```python
from build123d import *

# Parameters (mm, degrees)
SKETCH1_R                 = 4.7625
SKETCH1_W                 = 6.5278
SKETCH1_H                 = 6.5278
SKETCH1_H_2               = 6.348837221
BOSS_EXTRUDE1_DEPTH       = 6.35
F_6_CLEARANCE_HOLE1_D     = 3.7973
F_6_CLEARANCE_HOLE1_DEPTH = 12.7
F_6_CLEARANCE_HOLE1_TIP   = 1.140824014
SKETCH7_W                 = 6.35
SKETCH7_H                 = 6.1722
BOSS_EXTRUDE2_DEPTH       = 1.016
SKETCH8_W                 = 6.35
SKETCH8_H                 = 6.1722
BOSS_EXTRUDE3_DEPTH       = 1.016
SKETCH9_R                 = 1.5875
CUT_EXTRUDE1_DEPTH        = 161.894515133
CUT_EXTRUDE2_DEPTH        = 161.894515133


with BuildPart() as part:
    # Sketch1 → Boss-Extrude1 (new body)
    with BuildSketch(Plane(origin=(0, 0, 0), x_dir=(0, 0, -1), z_dir=(1, 0, 0))):
        Polygon((0, 0), (-14.664696837, 25.4), (-144.085303163, 25.4), (-158.75, 0), align=None)
        with Locations((-130.048, 12.7)):
            Circle(SKETCH1_R, mode=Mode.SUBTRACT)
        with Locations((-28.702, 12.7)):
            Circle(SKETCH1_R, mode=Mode.SUBTRACT)
        with Locations((-17.750796837, 12.6111)):
            Rectangle(SKETCH1_W, SKETCH1_H, mode=Mode.SUBTRACT)
        with Locations((-140.999203163, 12.70058139)):
            Rectangle(SKETCH1_W, SKETCH1_H_2, mode=Mode.SUBTRACT)
        with Locations((-79.4639, 12.7889)):
            Rectangle(SKETCH1_W, SKETCH1_H, mode=Mode.SUBTRACT)
    extrude(amount=BOSS_EXTRUDE1_DEPTH)

    # #6 Clearance Hole1
    with Locations(Plane(origin=(0, 25.4, 0), x_dir=(1, 0, 0), z_dir=(0, 1, 0))):
        with Locations((3.175, -79.375)):
            Hole(F_6_CLEARANCE_HOLE1_D / 2, depth=F_6_CLEARANCE_HOLE1_DEPTH)
            with Locations((0, 0, -(F_6_CLEARANCE_HOLE1_DEPTH + F_6_CLEARANCE_HOLE1_TIP / 2))):  # 118° drill point
                Cone(0, F_6_CLEARANCE_HOLE1_D / 2, F_6_CLEARANCE_HOLE1_TIP, mode=Mode.SUBTRACT)

    # Sketch7 → Boss-Extrude2 (add)
    with BuildSketch(Plane(origin=(0, 0, 0), x_dir=(-1, 0, 0), z_dir=(0, 0.499999999999998, -0.8660254037844397))):
        with Locations((-3.175, 19.893293675)):
            Rectangle(SKETCH7_W, SKETCH7_H)
    extrude(amount=BOSS_EXTRUDE2_DEPTH)

    # Sketch8 → Boss-Extrude3 (add)
    with BuildSketch(Plane(origin=(0, 68.740766425, 119.0625), x_dir=(1, 0, 0), z_dir=(0, 0.500000000000004, 0.8660254037844365))):
        with Locations((3.175, -59.481706325)):
            Rectangle(SKETCH8_W, SKETCH8_H)
    extrude(amount=BOSS_EXTRUDE3_DEPTH)

    # Sketch9 → Cut-Extrude1 (cut, through all)
    with BuildSketch(Plane(origin=(6.35, 0, 0), x_dir=(0, 0, -1), z_dir=(1, 0, 0))):
        with Locations((-151.13, 3.81)):
            Circle(SKETCH9_R)
        with Locations((-7.62, 3.81)):
            Circle(SKETCH9_R)
    extrude(amount=-CUT_EXTRUDE1_DEPTH, mode=Mode.SUBTRACT)

    # Sketch10 → Cut-Extrude2 (cut, through all)
    with BuildSketch(Plane(origin=(6.35, 0, 0), x_dir=(0, 0, -1), z_dir=(1, 0, 0))):
        Polygon((-90.0938, 7.366), (-90.0938, 17.550906382), (-115.628105199, 7.366), align=None)
        Polygon((-119.901628846, 7.849093618), (-94.367323648, 18.034), (-119.901628846, 18.034), align=None)
        Polygon((-68.834, 7.850665489), (-43.375663722, 18.034), (-68.834, 18.034), align=None)
        Polygon((-39.116, 7.366), (-39.116, 17.549334511), (-64.574336278, 7.366), align=None)
    extrude(amount=-CUT_EXTRUDE2_DEPTH, mode=Mode.SUBTRACT)


solid = part.part
```
Here's how the part is built. I have some questions about the finished solid (model axes, mm). A direction names the side the tool comes from. Coordinates: 2 decimals unless noted, no trailing zeros. Loops run counter-clockwise (first coordinate to the right, second up) from the corner with the lowest first, then second, coordinate; pieces in that order, holes last. Notation, with made-up numbers: (34.5, -18) - (50.5, -18) arc R28 cw to (50.5, 10) - close; hole circle Ø8 at (87.5, -39). An arc over 180 degrees is marked (long way). Return JSON: item names as keys, results as strings. Group by question number.
Item 1: If we section it at D-D on x = 2.25: State how many separate pieces and enclosed holes the cut face has, and give its area (3 significant figures).
Item 2: We'd pull the mould along Z, two halves only. Please class faces 1 (the face through (3.131, 7.176, 4.143)), 2 (the face through (3, 13, 76.2)), 3 (the face through (6.35, 7, 80)): +Z half, -Z half, draft (parallel to the pull), parting line (faces both ways), or undercut.
Item 3: Will these pins go through, and if not, where does the flat tip stop? P1, Ø3, axis at x = 3, z = 18.5, coming from the -Y side; P2, Ø1.9, axis at x = 4, y = 14, coming from the +Z side; P3, Ø3, axis at x = 2.5, y = 13, coming from the +Z side; P4, Ø3, axis at x = 2.5, y = 11.5, coming from the +Z side.
Item 4: If we section it at A-A on y = 3.81: Write out the boundary of the cut face in (x, z).
Item 5: On a 3-axis mill with a long thin cutter (end or side, diameter ignored), from which of +Z, -Z, +X, -X, +Y, -Y can I reach the whole of each face in a straight line? I mean faces 4 (the face through (5, 25.4, 78)), 5 (the face through (3, 7.366, 52)). Say none if no direction works.
Item 6: If we section it at B-B on z = 30.5: Write out the boundary of the cut face in (x, y).
Item 7: If we section it at C-C on z = 110: Write out the boundary of the cut face in (x, y).
Item 8: I need wall thicknesses on line 1 (Y direction, x = 1.5, z = 51.5); line 2 (Z direction, x = 6.25, y = 3.75); line 3 (Y direction, x = 2.5, z = 151.13). Which ranges of each line are inside material? Lowest first, please. Write a range as from..to.
Calculated:
{
 "1": {"separate pieces": "1", "enclosed holes": "10", "area": "2,840 mm^2"},
 "2": {"face 1": "-Z half", "face 2": "undercut", "face 3": "draft"},
 "3": {"P1": "stops at y = 0", "P2": "stops at z = 151.22", "P3": "stops at z = 152.11", "P4": "stops at z = 152.98"},
 "4": {"outline": "(0, 2.2) - (6.35, 2.2) - (6.35, 6.03) - (0, 6.03) - close; (0, 9.21) - (6.35, 9.21) - (6.35, 149.54) - (0, 149.54) - close; (0, 152.72) - (6.35, 152.72) - (6.35, 156.55) - (0, 156.55) - close"},
 "5": {"face 4": "+Z, -Z, +X, -X, +Y", "face 5": "+X, -X"},
 "6": {"outline": "(0, 0) - (6.35, 0) - (6.35, 8.29) - (0, 8.29) - close; (0, 17.11) - (6.35, 17.11) - (6.35, 25.4) - (0, 25.4) - close"},
 "7": {"outline": "(0, 0) - (6.35, 0) - (6.35, 7.37) - (0, 7.37) - close; (0, 9.61) - (6.35, 9.61) - (6.35, 11.8) - (0, 11.8) - close; (0, 18.03) - (6.35, 18.03) - (6.35, 25.4) - (0, 25.4) - close"},
 "8": {"line 1": "y = 0..7.37, 12.6..14.78, 18.03..25.4", "line 2": "z = 2.17..6.03, 9.21..149.54, 152.72..156.58", "line 3": "y = 0..2.22, 5.4..13.2, 15.01..15.23"}
}
